CAD build for the part. Positions are in the model's coordinates, mm. A direction names the side the tool comes from. Coordinates: 2 decimals unless noted, no trailing zeros. Write each loop counter-clockwise with the first axis right and the second up, starting at its lowest first coordinate (ties: lowest second). Pieces come first, ordered by that corner, then holes. Notation, with made-up numbers: (-38.75, 21.5) - (17.25, 21.5) arc R28 cw to (17.25, 57.5) - close; hole circle Ø10 at (46.5, 58.5). An arc over 180 degrees is marked (long way). Answer in a Markdown table with one row per item. Add a question column.
Q1. Two-plate mould, pull along X, no slides. Class faces 6 (the cylindrical face through (0, -2, 63)), 7 (the flat face through (-9, 0, 45.8)), 8 (the flat face through (-7, 10, 30.8)): +X half, -X half, draft (parallel to the pull), parting line (faces both ways), or undercut.
Q2. Pin check, flat tips, straight feed: pin 1 (0.8 mm diameter, centred on y = 12.5, z = -6.5, fed in from +X); pin 2 (1 mm diameter, centred on y = 6, z = 24, fed in from -X); pin 3 (3 mm diameter, centred on x = 1.5, y = 13, fed in from +Z). Stop position of each tip, or through.
Q3. Band-saw the part on C-C (y = 0). List the corners of the cut face in (x, z).
Q4. Band-saw the part on A-A (z = 53). List the corners of the cut face in (x, y), and give its area (3 significant figures).
Q5. Drill centre lines: line 1 along Y through (x, z) = (0, 49); line 2 along Z through (x, y) = (-5.75, 17.5); line 3 along Y through (x, z) = (-0.75, 55). Where is each one in solid material? Low to high. Write a range as from..to.
Q6. Band-saw the part on D-D (z = 39.5). List the corners of the cut face in (x, y).
Q7. 3-axis set-ups, long thin cutter, end or side, ignore diameter. For faces 1 (the cylindrical face through (0, -10, 51)), 2 (the flat face through (0, 0, 68.1)), 3 (the flat face through (0, 15, -7.468)), 4 (the flat face through (0, 1.5, 64)), 5 (the cylindrical face through (-11.99, 0.53, 15.18)): which of +Z, -Z, +X, -X, +Y, -Y reach the whole face in a straight line?
Q8. Band-saw the part on B-B (y = 14). List the corners of the cut face in (x, z), and give its area (3 significant figures).
```python
from build123d import *

# Parameters (mm, degrees)
SKETCH1_R           = 12
BOSS_EXTRUDE1_DEPTH = 30.8
SKETCH2_R           = 12.5
BOSS_EXTRUDE2_DEPTH = 25
SKETCH3_R           = 3.5
BOSS_EXTRUDE3_DEPTH = 2.5
SKETCH4_R           = 2
BOSS_EXTRUDE4_DEPTH = 9.8
CUT_EXTRUDE1_DEPTH  = 8.5
SKETCH6_R           = 11.75
BOSS_EXTRUDE5_DEPTH = 10.7
SKETCH7_W           = 18.699432978
SKETCH7_H           = 3
BOSS_EXTRUDE6_DEPTH = 20
SKETCH8_R           = 1.5
CUT_EXTRUDE2_DEPTH  = 10
SKETCH9_R           = 2
CUT_EXTRUDE3_DEPTH  = 10
SKETCH10_W          = 16.5
SKETCH10_H          = 1.5
CUT_EXTRUDE4_DEPTH  = 10


with BuildPart() as part:
    # Sketch1 → Boss-Extrude1 (new body)
    with BuildSketch(Plane.XY):
        Circle(SKETCH1_R)
    extrude(amount=BOSS_EXTRUDE1_DEPTH)

    # Sketch2 → Boss-Extrude2 (add)
    with BuildSketch(Plane.XY.offset(30.8)):
        Circle(SKETCH2_R)
    extrude(amount=BOSS_EXTRUDE2_DEPTH)

    # Sketch3 → Boss-Extrude3 (add)
    with BuildSketch(Plane.XY.offset(55.8)):
        Circle(SKETCH3_R)
    extrude(amount=BOSS_EXTRUDE3_DEPTH)

    # Sketch4 → Boss-Extrude4 (add)
    with BuildSketch(Plane.XY.offset(58.3)):
        Circle(SKETCH4_R)
    extrude(amount=BOSS_EXTRUDE4_DEPTH)

    # Sketch5 → Cut-Extrude1 (cut)
    with BuildSketch(Plane.XY.offset(68.1)):
        with BuildLine():
            Line((-1.322875656, 1.5), (0, 1.5))
            Line((0, 1.5), (1.322875656, 1.5))
            ThreePointArc((1.322875656, 1.5), (0, 2), (-1.322875656, 1.5))
        make_face()
    extrude(amount=-CUT_EXTRUDE1_DEPTH, mode=Mode.SUBTRACT)

    # Sketch6 → Boss-Extrude5 (add)
    with BuildSketch(Plane(origin=(0, 0, 0), x_dir=(-1, 0, 0), z_dir=(0, 0, -1))):
        Circle(SKETCH6_R)
    extrude(amount=BOSS_EXTRUDE5_DEPTH)

    # Sketch7 → Boss-Extrude6 (add)
    with BuildSketch(Plane(origin=(0, 0, 0), x_dir=(1, 0, 0), z_dir=(0, 1, 0))):
        with Locations((0, 6.81237414)):
            Rectangle(SKETCH7_W, SKETCH7_H)
    extrude(amount=BOSS_EXTRUDE6_DEPTH)

    # Sketch8 → Cut-Extrude2 (cut)
    with BuildSketch(Plane.XY.offset(55.8)):
        with Locations((0, -8.5)):
            Circle(SKETCH8_R)
    cut_extrude2 = extrude(amount=-CUT_EXTRUDE2_DEPTH, mode=Mode.SUBTRACT)

    # Mirror1: Cut-Extrude2 across plane
    add(cut_extrude2.mirror(Plane.ZX), mode=Mode.SUBTRACT)

    # Sketch9 → Cut-Extrude3 (cut)
    with BuildSketch(Plane.XY.offset(55.8)):
        with Locations((-8.5, 0)):
            Circle(SKETCH9_R)
    cut_extrude3 = extrude(amount=-CUT_EXTRUDE3_DEPTH, mode=Mode.SUBTRACT)

    # Mirror3: Cut-Extrude3 across plane
    add(cut_extrude3.mirror(Plane(origin=(0, 0, 0), x_dir=(0, 0, 1), z_dir=(1, 0, 0))), mode=Mode.SUBTRACT)

    # Sketch10 → Cut-Extrude4 (cut)
    with BuildSketch(Plane(origin=(0, 20, 0), x_dir=(1, 0, 0), z_dir=(0, 1, 0))):
        with Locations((0.137296408, 6.718389465)):
            Rectangle(SKETCH10_W, SKETCH10_H)
    extrude(amount=-CUT_EXTRUDE4_DEPTH, mode=Mode.SUBTRACT)


solid = part.part
```
Checked values:
| question | item | result |
|---|---|---|
| 1 | face 6 | parting line |
| 1 | face 7 | undercut |
| 1 | face 8 | draft |
| 2 | pin 1 | stops at x = 9.35 |
| 2 | pin 2 | stops at x = -10.67 |
| 2 | pin 3 | stops at z = 55.8 |
| 3 | outline | (-12.5, 30.8) - (-12, 30.8) - (-12, 0) - (-11.75, 0) - (-11.75, -10.7) - (11.75, -10.7) - (11.75, 0) - (12, 0) - (12, 30.8) - (12.5, 30.8) - (12.5, 55.8) - (10.5, 55.8) - (10.5, 45.8) - (6.5, 45.8) - (6.5, 55.8) - (3.5, 55.8) - (3.5, 58.3) - (2, 58.3) - (2, 68.1) - (-2, 68.1) - (-2, 58.3) - (-3.5, 58.3) - (-3.5, 55.8) - (-6.5, 55.8) - (-6.5, 45.8) - (-10.5, 45.8) - (-10.5, 55.8) - (-12.5, 55.8) - close |
| 4 | outline | circle Ø25 at (0, 0); hole circle Ø4 at (-8.5, 0); hole circle Ø3 at (0, -8.5); hole circle Ø3 at (0, 8.5); hole circle Ø4 at (8.5, 0) |
| 4 | area | 452 mm² |
| 5 | line 1 | y = -12.5..-10, -7..7, 10..12.5 |
| 5 | line 2 | z = -8.31..-7.47, -5.97..-5.31 |
| 5 | line 3 | y = -12.48..-9.8, -7.2..7.2, 9.8..12.48 |
| 6 | outline | circle Ø25 at (0, 0) |
| 7 | face 1 | +Z |
| 7 | face 2 | +Z, +X, -X, +Y, -Y |
| 7 | face 3 | +Y |
| 7 | face 4 | +Z, +X, -X, +Y |
| 7 | face 5 | none |
| 8 | outline | (-9.35, -8.31) - (9.35, -8.31) - (9.35, -5.31) - (-9.35, -5.31) - close; hole (-8.11, -7.47) - (8.39, -7.47) - (8.39, -5.97) - (-8.11, -5.97) - close |
| 8 | area | 31.3 mm² |
